from build123d import *

# Parameters (mm, degrees)
SKETCH1_R           = 95
BOSS_EXTRUDE1_DEPTH = 600
SHELL1_T            = 10
SKETCH2_R           = 30
BOSS_EXTRUDE2_DEPTH = 18
SKETCH4_R           = 20
BOSS_EXTRUDE3_DEPTH = 95


with BuildPart() as part:
    # Sketch1 → Boss-Extrude1 (new body)
    with BuildSketch(Plane(origin=(0, 0, 0), x_dir=(1, 0, 0), z_dir=(0, 1, 0))):
        Circle(SKETCH1_R)
    extrude(amount=BOSS_EXTRUDE1_DEPTH)

    # Shell1 (no face opened: a closed hollow body)
    add(offset(amount=-SHELL1_T, mode=Mode.PRIVATE), mode=Mode.SUBTRACT)

    # Sketch2 → Boss-Extrude2 (add)
    with BuildSketch(Plane(origin=(0, 0, -95), x_dir=(-1, 0, 0), z_dir=(0, 0, -1))):
        with BuildLine():
            Line((0, 0), (95, 0))
            Line((95, 0), (200, 0))
            ThreePointArc((200, 0), (268.163356789, 54.070254514), (231.023569289, 132.749805964))
            Line((231.023569289, 132.749805964), (95, 200))
            Line((95, 200), (0, 200))
            Line((0, 200), (0, 0))
        make_face()
        with Locations((200, 70)):
            Circle(SKETCH2_R, mode=Mode.SUBTRACT)
        with BuildLine():
            Line((0, 600), (95, 600))
            Line((95, 600), (170, 600))
            ThreePointArc((170, 600), (226.448348767, 560.336762809), (208.265889327, 493.786130718))
            Line((208.265889327, 493.786130718), (95, 400))
            Line((95, 400), (0, 400))
            Line((0, 400), (0, 600))
        make_face()
    boss_extrude2 = extrude(amount=-BOSS_EXTRUDE2_DEPTH)

    # Mirror1: Boss-Extrude2 across plane
    add(boss_extrude2.mirror(Plane(origin=(0, 0, 0), x_dir=(1, 0, 0), z_dir=(0, 0, -1))))

    # Sketch4 → Boss-Extrude3 (add, symmetric)
    with BuildSketch(Plane.XY):
        with Locations((-170, 540)):
            Circle(SKETCH4_R)
    extrude(amount=BOSS_EXTRUDE3_DEPTH, both=True)


solid = part.part
Work out the finished part from the listing and answer in its coordinate system (mm). A direction names the side the tool comes from. Round coordinates to 2 decimals unless told otherwise and drop trailing zeros. Loops run counter-clockwise (first coordinate to the right, second up) from the corner with the lowest first, then second, coordinate; pieces in that order, holes last. Notation, with made-up numbers: (48.25, -26.75) - (53.25, -26.75) arc R25 ccw to (53.25, 1.25) - close; hole circle Ø8 at (3.25, 66). An arc over 180 degrees is marked (long way). Use one line per item in the form item = value. Start each with the question number.
(1) Consider line 1 (Y direction, x = 8, z = -15.5); line 2 (Y direction, x = -200, z = -82); line 3 (Z direction, x = -9, y = 447). Determine where each line is inside the solid, lowest interval first.
(2) Find section A-A on z = 9. Determine the outline of the cut face in (x, y).
(3) Find section C-C on y = 540. Determine the outline of the cut face in (x, z), and give its area (3 significant figures).
(4) Which of the six approach directions +Z, -Z, +X, -X, +Y, -Y give full straight-line access (tool end or side, diameter ignored) to faces 4 (the face through (-1, 590, -1)), 5 (the face through (-103, 101, 95)), 6 (the face through (-69, 400, -88)), 7 (the face through (-152.426, 447.55, -86.126))?
(5) Flat-ended cylindrical pins translate along their axes: P1, Ø6.5, axis at y = 69.5, z = 82, coming from the +X side; P2, Ø6.5, axis at y = 98.5, z = -80.5, coming from the +X side; P3, Ø8, axis at y = 91, z = 8, coming from the +X side. Find the tip coordinate at first contact, or state that the pin passes through.
(6) Find section D-D on x = -12.5. Determine the outline of the cut face in (y, z), and give its area (3 significant figures).
(7) Find section B-B on x = -141. Determine the outline of the cut face in (y, z).
(8) Determine the mould class of faces 1 (the face through (81.075, 295.94, -25.532)), 2 (the face through (-138, 79, 77)), 3 (the face through (-267.85, 52.79, -86.13)) for opening direction Y: +Y half, -Y half, draft (parallel to the pull), parting line (faces both ways), or undercut.
Answer list:
q1.line_1 = 0 to 10, 590 to 600
q1.line_2 = 0 to 40, 100 to 148.09, 486.94 to 591.96
q1.line_3 = -95 to -77, 77 to 95
q2.outline = circle Ø40 at (-170, 540); (-94.57, 0) - (94.57, 0) - (94.57, 600) - (-94.57, 600) - close; hole (-84.52, 10) - (84.52, 10) - (84.52, 590) - (-84.52, 590) - close
q3.outline = (-230, -95) - (0, -95) arc R95 ccw to (0, 95) - (-230, 95) - (-230, 77) - (-190, 77) - (-190, -77) - (-230, -77) - close; hole (-150, -77) - (-55.64, -77) arc R95 cw to (-55.64, 77) - (-150, 77) - close; hole (-36, -77) - (0, -77) - (0, -85) arc R85 ccw to (0, 85) - (0, 77) - (-36, 77) arc R85 ccw to start
q3.area = 19,100 mm^2
q4.face_4 = none
q4.face_5 = +Z, +X, -X, +Y, -Y
q4.face_6 = -Z, -X
q4.face_7 = +Z, -Z, -X
q5.P1 = 53.14
q5.P2 = 55.29
q5.P3 = 94.92
q6.outline = (0, -95) - (200, -95) - (200, -94.17) - (400, -94.17) - (400, -95) - (600, -95) - (600, 95) - (400, 95) - (400, 94.17) - (200, 94.17) - (200, 95) - (0, 95) - close; hole (10, -77) - (200, -77) - (200, -84.08) - (400, -84.08) - (400, -77) - (590, -77) - (590, 77) - (400, 77) - (400, 84.08) - (200, 84.08) - (200, 77) - (10, 77) - close
q6.area = 21,500 mm^2
q7.outline = (0, -95) - (177.26, -95) - (177.26, -77) - (0, -77) - close; (0, 77) - (177.26, 77) - (177.26, 95) - (0, 95) - close; (438.09, -95) - (600, -95) - (600, -77) - (438.09, -77) - close; (438.09, 77) - (600, 77) - (600, 95) - (438.09, 95) - close
q8.face_1 = undercut
q8.face_2 = draft
q8.face_3 = parting line
